```python
from build123d import *

# Parameters (mm, degrees)
SKETCH_1_R               = 16.5
EXTRUDE_1_DEPTH          = 6
EXTRUDE_START            = -6
EXTRUDE_2_DEPTH          = 6
EXTRUDE_3_DEPTH          = 21
SKETCH_4_R               = 3.5
CUT_EXTRUDE_1_DEPTH      = 47.608743815
CUT_EXTRUDE_3_DEPTH      = 53.832281798
CUT_EXTRUDE_3_DEPTH_BACK = 53.832281798
EXTRUDE_4_DEPTH          = 21
FILLET_3_R               = 10


with BuildPart() as part:
    # 草图1 → 凸台-拉伸1 (new body)
    with BuildSketch(Plane.XY):
        Circle(SKETCH_1_R)
        Polygon((13.35, 0), (9.439875529, -9.439875529), (0, -13.35), (-9.439875529, -9.439875529), (-13.35, 0), (-9.439875529, 9.439875529), (0, 13.35), (9.439875529, 9.439875529), align=None, mode=Mode.SUBTRACT)
    extrude(amount=EXTRUDE_1_DEPTH)

    # 草图2 → 凸台-拉伸2 (add)
    with BuildSketch(Plane.XY.offset(6).offset(EXTRUDE_START)):
        with BuildLine():
            Line((-10.5, -12.727922061), (-10.5, -30))
            Line((-10.5, -30), (10.5, -30))
            Line((10.5, -30), (10.5, -12.727922061))
            ThreePointArc((10.5, -12.727922061), (0, -16.5), (-10.5, -12.727922061))
        make_face()
    extrude(amount=EXTRUDE_2_DEPTH)

    # 草图3 → 凸台-拉伸3 (add)
    with BuildSketch(Plane(origin=(10.5, 0, 0), x_dir=(0, 0, -1), z_dir=(1, 0, 0))):
        Polygon((-6, -24), (-9.742640687, -24), (-15.742640687, -30), (-7.257359313, -30), (-6, -28.742640687), align=None)
        Polygon((-6, -30), (-6, -28.742640687), (-7.257359313, -30), align=None)
        Polygon((-7.257359313, -30), (-15.742640687, -30), (-21.5, -35.757359313), (-17.257359313, -40), align=None)
    extrude(amount=-EXTRUDE_3_DEPTH)

    # 草图4 → 切除-拉伸1 (cut, through all)
    with BuildSketch(Plane(origin=(0, -7.128679656, -7.128679656), x_dir=(1, 0, 0), z_dir=(0, 0.7071067811865438, 0.7071067811865513))):
        with Locations(Location((0, -34.487067043, 0), (0, 0, 270))):
            Circle(SKETCH_4_R)
    extrude(amount=-CUT_EXTRUDE_1_DEPTH, mode=Mode.SUBTRACT)

    # 草图5 → 切除-拉伸3 (cut, two sides: drawn at the far end of the back side and taken through both)
    with BuildSketch(Plane(origin=(10.5, 0, 0), x_dir=(0, 0, -1), z_dir=(1, 0, 0)).offset(-CUT_EXTRUDE_3_DEPTH_BACK)):
        Polygon((0, -22.742640687), (-7.257359313, -30), (0, -30), align=None)
    extrude(amount=CUT_EXTRUDE_3_DEPTH + CUT_EXTRUDE_3_DEPTH_BACK, mode=Mode.SUBTRACT)

    # 草图6 → 凸台-拉伸4 (add)
    with BuildSketch(Plane(origin=(10.5, 0, 0), x_dir=(0, 0, -1), z_dir=(1, 0, 0))):
        Polygon((-6, -20.257359313), (-9.742640687, -24), (-6, -24), align=None)
    extrude(amount=-EXTRUDE_4_DEPTH)

    # 圆角3
    fillet_3_edges = [part.edges().sort_by_distance(p)[0] for p in [
        (-10.5, -12.727922061, 3),
        (10.5, -12.727922061, 3),
        (-10.5, -37.878679656, 19.378679656),
        (10.5, -37.878679656, 19.378679656),
    ]]
    fillet(fillet_3_edges, radius=FILLET_3_R)


solid = part.part
```
Geometry check sheet. Reference: the model listing, model coordinates, mm. A direction names the side the tool comes from. Round coordinates to 2 decimals unless told otherwise and drop trailing zeros. Loops run counter-clockwise (first coordinate to the right, second up) from the corner with the lowest first, then second, coordinate; pieces in that order, holes last. Notation, with made-up numbers: (81.25, -32) -> (135.25, -32) arc R20 ccw to (135.25, -28) -> close; hole circle Ø4 at (37, -5.75). An arc over 180 degrees is marked (long way). Use a Markdown table: item, result.
(1) Sectioned sample at C-C (y = 8.5). Enter the section's corners in (x, z), then the cut area to 3 significant figures.
Calculated:
| item | result |
|---|---|
| outline | (-14.14, 0) -> (-9.83, 0) -> (-9.83, 6) -> (-14.14, 6) -> close; (9.83, 0) -> (14.14, 0) -> (14.14, 6) -> (9.83, 6) -> close |
| area | 51.8 mm² |
(2) Sectioned sample at A-A (x = 8). Enter the section's corners in (y, z).
Calculated:
| item | result |
|---|---|
| outline | (-37.61, 14.86) -> (-22.74, 0) -> (-10.04, 0) -> (-10.04, 6) -> (-20.26, 6) -> (-33.36, 19.11) -> close; (10.04, 0) -> (14.43, 0) -> (14.43, 6) -> (10.04, 6) -> close |
(3) Go/stop test with flat-tipped pins: P1, Ø1.5, axis at x = 8, y = -29, coming from the +Z side; P2, Ø4, axis at x = 9.5, z = 5, coming from the -Y side; P3, Ø10, axis at x = 9, z = 8.5, coming from the -Y side. Record where each tip stops, or that it passes through.
Calculated:
| item | result |
|---|---|
| P1 | z = 15.49 |
| P2 | y = -29.74 |
| P3 | y = -36.24 |
(4) Set-up check for faces 5 (the flat face through (0, -14, 6)), 6 (the flat face through (11.422, -4.654, 2.958)), 7 (the flat face through (10.5, -25, 6)): record each of +Z, -Z, +X, -X, +Y, -Y from which the full face is reachable in a straight line by a thin tool's end or side.
Calculated:
| item | result |
|---|---|
| face 5 | +Z, +X, -X, +Y |
| face 6 | +Z, -Z |
| face 7 | +Z, -Z, +X, -Y |
(5) Mould release check, pull along Y, two halves, no side actions. Record for faces 1 (the flat face through (0.15, -26.18, 11.92)), 2 (the flat face through (-10.5, -25, 6)), 3 (the flat face through (-0.15, -29.33, 6.59)), 4 (the flat face through (-11.422, 4.654, 2.958)): released by +Y, released by -Y, zero draft, split by the parting line, or undercut.
Calculated:
| item | result |
|---|---|
| face 1 | released by +Y |
| face 2 | zero draft |
| face 3 | released by -Y |
| face 4 | undercut |
(6) Sectioned sample at D-D (x = -1.5). Enter the section's corners in (y, z).
Calculated:
| item | result |
|---|---|
| outline | (-39.96, 17.22) -> (-37.99, 15.25) -> (-33.75, 19.49) -> (-35.72, 21.46) -> close; (-33.52, 10.78) -> (-22.74, 0) -> (-12.73, 0) -> (-12.73, 6) -> (-20.26, 6) -> (-29.28, 15.02) -> close; (12.73, 0) -> (16.43, 0) -> (16.43, 6) -> (12.73, 6) -> close |
(7) Scan lines: probe 1 along X at (y, z) = (-28, 7.25); probe 2 along X at (y, z) = (-31, 14.5); probe 3 along X at (y, z) = (4, 3.25). Record each from-to range of solid material in increasing order.
Calculated:
| item | result |
|---|---|
| probe 1 | -10.5 to 10.5 |
| probe 2 | -10.36 to -2.63, 2.63 to 10.36 |
| probe 3 | -16.01 to -11.69, 11.69 to 16.01 |
(8) Sectioned sample at B-B (z = 3). Enter the section's corners in (x, y).
Calculated:
| item | result |
|---|---|
| outline | (-12.76, -10.46) arc R10 cw to (-10.5, -16.79) -> (-10.5, -25.74) -> (10.5, -25.74) -> (10.5, -16.79) arc R10 cw to (12.76, -10.46) arc R16.5 ccw (long way) to start; hole (-13.35, 0) -> (-9.44, -9.44) -> (0, -13.35) -> (9.44, -9.44) -> (13.35, 0) -> (9.44, 9.44) -> (0, 13.35) -> (-9.44, 9.44) -> close |
